CAD build for the part. Positions are in the model's coordinates, mm. A direction names the side the tool comes from. Round coordinates to 2 decimals unless told otherwise and drop trailing zeros. Loops run counter-clockwise (first coordinate to the right, second up) from the corner with the lowest first, then second, coordinate; pieces in that order, holes last. Notation, with made-up numbers: (73, -9.5) - (104, -9.5) arc R16 ccw to (104, -0.5) - close; hole circle Ø5 at (-0.5, 33.25). An arc over 180 degrees is marked (long way). One line per question, with ' | ' between items.
Autodesk Inventor part; units mm, degrees
ref_plane "YZ Plane" through (0, 0, 0) normal (1, 0, 0) x (0, 1, 0)
ref_plane "XZ Plane" through (0, 0, 0) normal (0, 1, 0) x (-1, 0, 0)
ref_plane "XY Plane" through (0, 0, 0) normal (0, 0, 1) x (1, 0, 0)
sketch "Sketch1" plane through (0, 0, 0) normal (0, 1, 0) x (-1, 0, 0)
  line L0 (26.6795, -25.7407) -> (-13.3205, -25.7407)
  line L1 (-13.3205, -25.7407) -> (-13.3205, -47.7407)
  line L2 (-13.3205, -47.7407) -> (26.6795, -47.7407)
  line L3 (26.6795, -47.7407) -> (26.6795, -25.7407)
  dimension "d0" = 40
  dimension "d1" = 22
extrude "Extrusion1" add sketch "Sketch1" along normal blind 8.5
sketch "Sketch2" plane through (0, 8.5, 0) normal (0, 1, 0) x (1, 0, 0)
  line L0 (13.3205, 25.7407) -> (13.3205, 47.7407)
  line L1 (13.3205, 47.0907) -> (3.3205, 47.0907)
  line L2 (3.3205, 47.0907) -> (3.3205, 26.3907)
  line L3 (3.3205, 26.3907) -> (13.3205, 26.3907)
  line L4 (13.3205, 26.3907) -> (13.3205, 47.0907)
  line L5 (13.3205, 47.7407) -> (-26.6795, 47.7407)
  line L6 (-26.6795, 25.7407) -> (13.3205, 25.7407)
  point P0 (13.3205, 26.3907)
  point P1 (8.3205, 47.0907)
  dimension "d6" = 10
  dimension "d23" = 0.65
  dimension "d24" = 0.65
extrude "Extrusion2" cut sketch "Sketch2" against normal blind 7.85
sketch "Sketch3" plane through (3.3205, 8.5, -26.3907) normal (1, 0, 0) x (0, 0, -1)
  line L0 (0.35, -4.25) -> (20.35, -4.25)
  line L1 (20.35, -4.25) -> (20.35, -5.85)
  line L2 (20.35, -5.85) -> (0.35, -5.85)
  line L3 (0.35, -5.85) -> (0.35, -4.25)
  line L4 (20.35, -5.05) -> (20.7, -5.05) construction
  line L5 (20.7, 0) -> (20.7, -7.85) construction
  line L6 (0.35, -5.05) -> (0, -5.05) construction
  line L7 (0, -7.85) -> (0, 0) construction
  line L8 (20.7, -7.85) -> (0, -7.85) construction
  dimension "d9" = 1.6
  dimension "d10" = 2
  dimension "d25" = 20
extrude "Extrusion3" add sketch "Sketch3" along normal up to surface (10 mm away)
sketch "Sketch4" plane through (3.3205, 4.25, -26.7407) normal (0, 1, 0) x (1, 0, 0)
  line L0 (0, 0) -> (10, 0)
  line L1 (10, 0) -> (10, 20)
  point P0 (-3.3205, -26.7407)
  point P1 (6.19, 2.5)
  dimension "d13" = 2.5
  dimension "d26" = 3.81
hole "Hole1" at (9.5105, 4.25, -29.2407) direction (0, -1, 0) diameter 1 depth 1.6
sketch "Sketch5" plane through (0, 8.5, 0) normal (0, 1, 0) x (1, 0, 0)
  line L0 (-26.3216, 47.7407) -> (3.3205, 47.7407) construction
  line L1 (3.3205, 47.7407) -> (3.3205, 25.7407) construction
  line L2 (3.3205, 25.7407) -> (-26.3216, 25.7407) construction
  line L3 (-26.3216, 25.7407) -> (-26.3216, 47.7407) construction
  line L4 (13.3205, 47.7407) -> (-26.6795, 47.7407)
  line L5 (3.3205, 26.3907) -> (3.3205, 47.0907)
  point P0 (3.3205, 36.7407)
decal "Decal1"
properties part number "Flysky FS-iA6 Receiver"
(1) Drop a flat-ended pin along its axis: P1, Ø3, axis at x = 9, z = -37, coming from the +Y side. Give the stop position or say it passes through.
Results found:
P1: stops at y = 4.25
(2) Probe L1, parallel to Y at x = 10, z = -44; L2, parallel to Z at x = 3.5, y = 1.5; L3, parallel to X at y = 3.5, z = -29.25. List the from-to ranges inside material, lowest first.
Results found:
L1: y = 0 to 0.65, 2.65 to 4.25 | L2: z = -47.74 to -47.09, -26.39 to -25.74 | L3: x = -26.68 to 9.01, 10.01 to 13.32
(3) Cut at C-C, the plane z = -29.25. Write the cut outline in (x, y).
Results found:
outline: (-26.68, 0) - (13.32, 0) - (13.32, 0.65) - (3.32, 0.65) - (3.32, 2.65) - (9.01, 2.65) - (9.01, 4.25) - (3.32, 4.25) - (3.32, 8.5) - (-26.68, 8.5) - close; (10.01, 2.65) - (13.32, 2.65) - (13.32, 4.25) - (10.01, 4.25) - close
(4) Cut at A-A, the plane z = -33. Write the cut outline in (x, y).
Results found:
outline: (-26.68, 0) - (13.32, 0) - (13.32, 0.65) - (3.32, 0.65) - (3.32, 2.65) - (13.32, 2.65) - (13.32, 4.25) - (3.32, 4.25) - (3.32, 8.5) - (-26.68, 8.5) - close
(5) Cut at B-B, the plane y = 6. Write the cut outline in (x, z), then the cut area to 3 significant figures.
Results found:
outline: (-26.68, -47.74) - (13.32, -47.74) - (13.32, -47.09) - (3.32, -47.09) - (3.32, -26.39) - (13.32, -26.39) - (13.32, -25.74) - (-26.68, -25.74) - close | area: 673 mm²
(6) Two-plate mould, pull along Y, no slides. Class faces 1 (the face through (-26.68, 4, -37)), 2 (the face through (-6, 0, -37)), 3 (the face through (-11, 8.5, -37)), 4 (the face through (8, 0.65, -37)): released by +Y, released by -Y, zero draft, split by the parting line, or undercut.
Results found:
face 1: zero draft | face 2: released by -Y | face 3: released by +Y | face 4: undercut
(7) Tool access for faces 5 (the face through (9.7, 3.44, -28.78)), 6 (the face through (-6, 4, -47.741)), 7 (the face through (8, 2.65, -37)), 8 (the face through (8, 5, -26.391)): list every direction of +Z, -Z, +X, -X, +Y, -Y with a clear straight run to the whole face (end or side of a thin tool).
Results found:
face 5: +Y | face 6: -Z, +X, -X, +Y, -Y | face 7: +X | face 8: +X, +Y
